Build history of the part. All positions in model axes, mm. A direction names the side the tool comes from. Round coordinates to 2 decimals unless told otherwise and drop trailing zeros. Loops run counter-clockwise (first coordinate to the right, second up) from the corner with the lowest first, then second, coordinate; pieces in that order, holes last. Notation, with made-up numbers: (8, 88.5) - (29, 88.5) arc R19 cw to (29, 92.5) - close; hole circle Ø2 at (12, 3.5). An arc over 180 degrees is marked (long way). Use a Markdown table: item, result.
from build123d import *

# Parameters (mm, degrees)
BASPROSKE_W        = 7
BASPROSKE_H        = 8
TOOTHCUT_DEPTH     = 14.304134696
TEETHCUTS_COUNT    = 14
TEETHCUTS_ANGLE    = 334.285714286
BORSKE_R           = 2.5
BORE_DEPTH         = 50.0000508
CUT_EXTRUDE2_DEPTH = 10
SKETCH2_R          = 4.15
CUT_EXTRUDE3_DEPTH = 14.210255756


with BuildPart() as part:
    # BasProSke → Base-Revolve (revolve)
    with BuildSketch(Plane(origin=(0, 0, 0), x_dir=(1, 0, 0), z_dir=(0, 1, 0)), mode=Mode.PRIVATE) as base_revolve_sk:
        with Locations((3.5, 4)):
            Rectangle(BASPROSKE_W, BASPROSKE_H)
    revolve(base_revolve_sk.sketch.rotate(Axis((-10, 0, 0), (1, 0, 0)), 180), axis=Axis((-10, 0, 0), (1, 0, 0)))

    # TooCutSke → ToothCut (cut, through all)
    with BuildSketch(Plane(origin=(0, 0, 0), x_dir=(0, 0, -1), z_dir=(1, 0, 0))):
        with BuildLine():
            ThreePointArc((0.540393256, 5.723545765), (0, 5.749), (-0.540393256, 5.723545765))
            ThreePointArc((-0.540393256, 5.723545765), (-0.832220085, 6.912663993), (-1.603550271, 7.863566092))
            ThreePointArc((-1.603550271, 7.863566092), (0, 8.0254), (1.603550271, 7.863566092))
            ThreePointArc((1.603550271, 7.863566092), (0.832220085, 6.912663993), (0.540393256, 5.723545765))
        make_face()
    toothcut = extrude(amount=TOOTHCUT_DEPTH, mode=Mode.SUBTRACT)

    # TeethCuts: ToothCut ×14 about axis
    teethcuts_axis = Axis((-10, 0, 0), (1, 0, 0))
    for i in range(1, TEETHCUTS_COUNT):
        add(toothcut.rotate(teethcuts_axis, i * TEETHCUTS_ANGLE / (TEETHCUTS_COUNT - 1)), mode=Mode.SUBTRACT)

    # BorSke → Bore (cut, symmetric)
    with BuildSketch(Plane(origin=(0, 0, 0), x_dir=(0, 0, -1), z_dir=(1, 0, 0))):
        with Locations(Location((0, 0, 0), (0, 0, 180))):
            Circle(BORSKE_R)
    extrude(amount=BORE_DEPTH, both=True, mode=Mode.SUBTRACT)

    # Sketch1 → Cut-Extrude2 (cut)
    with BuildSketch(Plane(origin=(7, 0, 0), x_dir=(0, 0, -1), z_dir=(1, 0, 0))):
        with BuildLine():
            Line((3.872983346, 1), (4.75, 1))
            Line((4.75, 1), (4.75, -1))
            Line((4.75, -1), (3.872983346, -1))
            ThreePointArc((3.872983346, -1), (0, -4), (-3.872983346, -1))
            Line((-3.872983346, -1), (-4.75, -1))
            Line((-4.75, -1), (-4.75, 1))
            Line((-4.75, 1), (-3.872983346, 1))
            ThreePointArc((-3.872983346, 1), (0, 4), (3.872983346, 1))
        make_face()
    extrude(amount=-CUT_EXTRUDE2_DEPTH, mode=Mode.SUBTRACT)

    # Sketch2 → Cut-Extrude3 (cut, through all)
    with BuildSketch(Plane(origin=(7, 0, 0), x_dir=(0, 0, -1), z_dir=(1, 0, 0))):
        Circle(SKETCH2_R)
    extrude(amount=-CUT_EXTRUDE3_DEPTH, mode=Mode.SUBTRACT)


solid = part.part
Q1. Probe line 1 (Z direction, x = 1.75, y = 3.5); line 2 (Z direction, x = 1.75, y = 3.25); line 3 (Y direction, x = 6.25, z = -7.25). List the from-to ranges inside material, lowest first.
Results found:
| item | result |
|---|---|
| line 1 | z = -7.19 to -5.42, -4.56 to -2.23, 2.23 to 4.56, 5.42 to 7.19 |
| line 2 | z = -7.28 to -4.96, -4.74 to -2.58, 2.58 to 4.74, 4.96 to 7.28 |
| line 3 | y = -3.38 to -3.2, -0.63 to 0.63, 3.2 to 3.38 |
Q2. Cut at C-C, the plane z = 6.75. List the corners of the cut face in (x, y), plus the area to 3 significant figures.
Results found:
| item | result |
|---|---|
| outline | (0, -3.71) - (7, -3.71) - (7, -2.53) - (0, -2.53) - close; (0, -0.76) - (7, -0.76) - (7, 0.76) - (0, 0.76) - close; (0, 2.53) - (7, 2.53) - (7, 3.71) - (0, 3.71) - close |
| area | 27.3 mm2 |
Q3. Cut at B-B, the plane y = 2. List the corners of the cut face in (x, z), plus the area to 3 significant figures.
Results found:
| item | result |
|---|---|
| outline | (0, -6.01) - (7, -6.01) - (7, -3.64) - (0, -3.64) - close; (0, 3.64) - (7, 3.64) - (7, 6.01) - (0, 6.01) - close |
| area | 33.2 mm2 |
Q4. Drop flat-ended pins along their axis: pin 1 (1.5 mm diameter, centred on x = 1.5, y = -2, fed in from -Z); pin 2 (2 mm diameter, centred on x = 5, y = 5.5, fed in from -Z); pin 3 (3 mm diameter, centred on x = 5, z = 6, fed in from -Y). Give the stop position or say it passes through.
Results found:
| item | result |
|---|---|
| pin 1 | stops at z = -6.95 |
| pin 2 | stops at z = -5.15 |
| pin 3 | stops at y = -6.38 |
Q5. Cut at A-A, the plane z = 2.5. List the corners of the cut face in (x, y), plus the area to 3 significant figures.
Results found:
| item | result |
|---|---|
| outline | (0, -5.18) - (7, -5.18) - (7, -3.31) - (0, -3.31) - close; (0, 3.31) - (7, 3.31) - (7, 5.18) - (0, 5.18) - close |
| area | 26.1 mm2 |
Q6. Cut at D-D, the plane z = -4.5. List the corners of the cut face in (x, y).
Results found:
| item | result |
|---|---|
| outline | (0, -6.28) - (7, -6.28) - (7, -4.35) - (0, -4.35) - close; (0, -3.58) - (7, -3.58) - (7, -1) - (0, -1) - close; (0, 1) - (7, 1) - (7, 3.58) - (0, 3.58) - close; (0, 4.35) - (7, 4.35) - (7, 6.28) - (0, 6.28) - close |
Q7. Which spindle directions (+Z, -Z, +X, -X, +Y, -Y) get a long thin tool onto all of the face, cutting with end or side? Do faces 4 (the face through (3.451, 2.35, 6.555)), 5 (the face through (3.451, -5.846, -3.723)), 6 (the face through (3.45, 4.93, -4.87)), 7 (the face through (3.45, 5.87, -3.75)). Say none if no direction does.
Results found:
| item | result |
|---|---|
| face 4 | +Z, +X, -X |
| face 5 | +X, -X, -Y |
| face 6 | -Z, +X, -X |
| face 7 | +X, -X, +Y |
Q8. Pull direction Y, two halves, no side cores. Call faces 1 (the face through (0, 3.4, -3.4)), 2 (the face through (3.45, -6.91, 0.83)), 3 (the face through (3.55, -4.15, 0.08)): pulls with the +Y half, pulls with the -Y half, needs draft (parallel to the pull), parting line crosses it, or undercut.
Results found:
| item | result |
|---|---|
| face 1 | needs draft |
| face 2 | pulls with the -Y half |
| face 3 | undercut |
